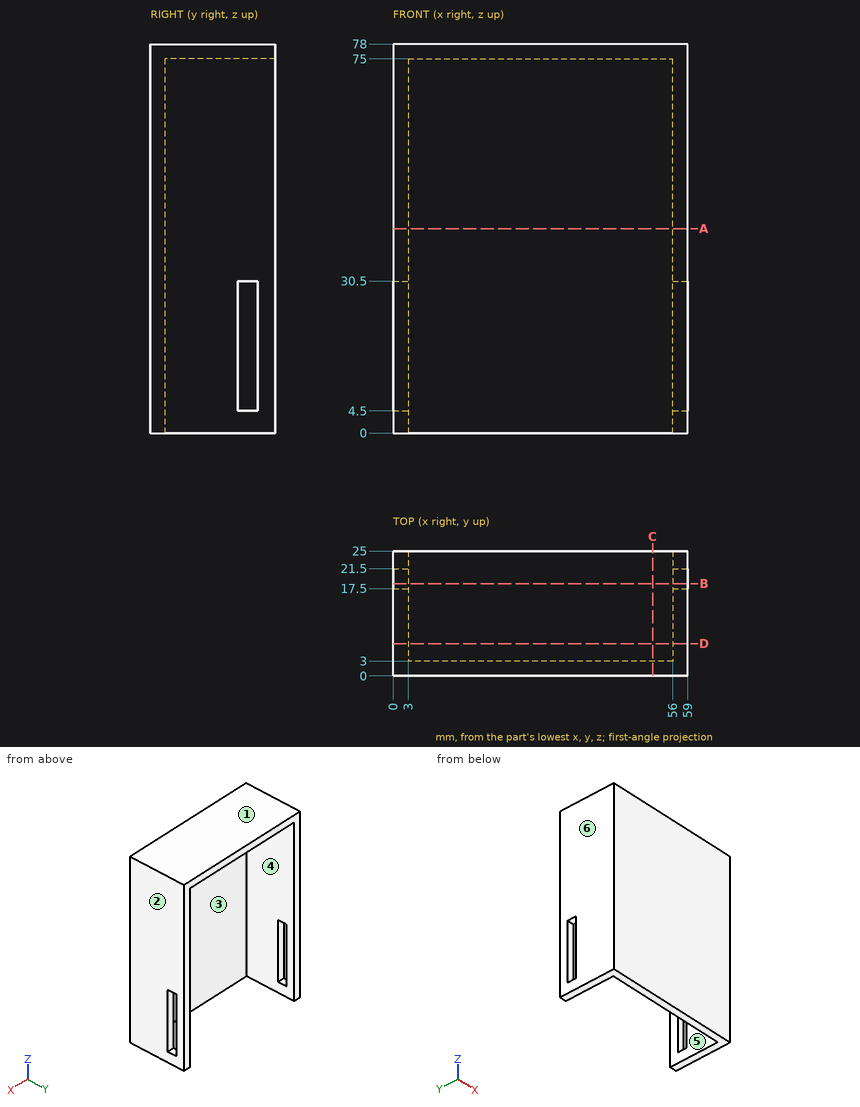
Job drawing, mm, ordinate dimensions from the low corner. One solid piece. A direction names the side the tool comes from. Coordinates: 2 decimals unless noted, no trailing zeros. Loops run counter-clockwise (first coordinate to the right, second up) from the corner with the lowest first, then second, coordinate; pieces in that order, holes last. Notation, with made-up numbers: (14, 53) - (42, 53) arc R20 cw to (42, 84) - close; hole circle Ø5 at (-26, -19.5). An arc over 180 degrees is marked (long way). Answer as a JSON object with one key per item and string values. Group by question number.
(1) Cut at A-A (z = 41). Give the cut face in (x, y), then the cut area to 3 significant figures.
(2) Cut at C-C (x = 52). Give the cut face in (y, z).
(3) Flat gauge pins, fed straight in: pin 1 (0.9 mm diameter, centred on x = 57, z = 24, fed in from -Y); pin 2 (5 mm diameter, centred on x = 16, z = 15, fed in from +Y); pin 3 (1.5 mm diameter, centred on x = 25.5, y = 5.5, fed in from -Z). Where does each tip first touch, or does it go through?
(4) Cut at B-B (y = 18.5). Give the cut face in (x, z).
(5) Probe line 1 along X through (y, z) = (12.25, 11); line 2 along Z through (x, y) = (37, 3.5); line 3 along Y through (x, z) = (34.5, 8.5). List the from-to ranges inside material, lowest first.
(6) Two-plate mould, pull along X, no slides. Class the marked faces 1, 2, 3 and 4: released by +X, released by -X, zero draft, split by the parting line, or undercut.
(7) Tool access for the marked faces 5 and 6: list every direction of +Z, -Z, +X, -X, +Y, -Y with a clear straight run to the whole face (end or side of a thin tool).
(8) Cut at D-D (y = 6.5). Give the cut face in (x, z), then the cut area to 3 significant figures.
Geometry says:
{
 "1": {"outline": "(0, 0) - (59, 0) - (59, 25) - (56, 25) - (56, 3) - (3, 3) - (3, 25) - (0, 25) - close", "area": "309 mm^2"},
 "2": {"outline": "(0, 0) - (3, 0) - (3, 75) - (25, 75) - (25, 78) - (0, 78) - close"},
 "3": {"pin 1": "stops at y = 0", "pin 2": "stops at y = 3", "pin 3": "stops at z = 75"},
 "4": {"outline": "(0, 0) - (3, 0) - (3, 4.5) - (0, 4.5) - close; (0, 30.5) - (3, 30.5) - (3, 75) - (56, 75) - (56, 30.5) - (59, 30.5) - (59, 78) - (0, 78) - close; (56, 0) - (59, 0) - (59, 4.5) - (56, 4.5) - close"},
 "5": {"line 1": "x = 0 to 3, 56 to 59", "line 2": "z = 75 to 78", "line 3": "y = 0 to 3"},
 "6": {"face 1": "zero draft", "face 2": "released by +X", "face 3": "undercut", "face 4": "undercut"},
 "7": {"face 5": "-Z, +Y", "face 6": "+Z, -Z, -X, +Y, -Y"},
 "8": {"outline": "(0, 0) - (3, 0) - (3, 75) - (56, 75) - (56, 0) - (59, 0) - (59, 78) - (0, 78) - close", "area": "627 mm^2"}
}
